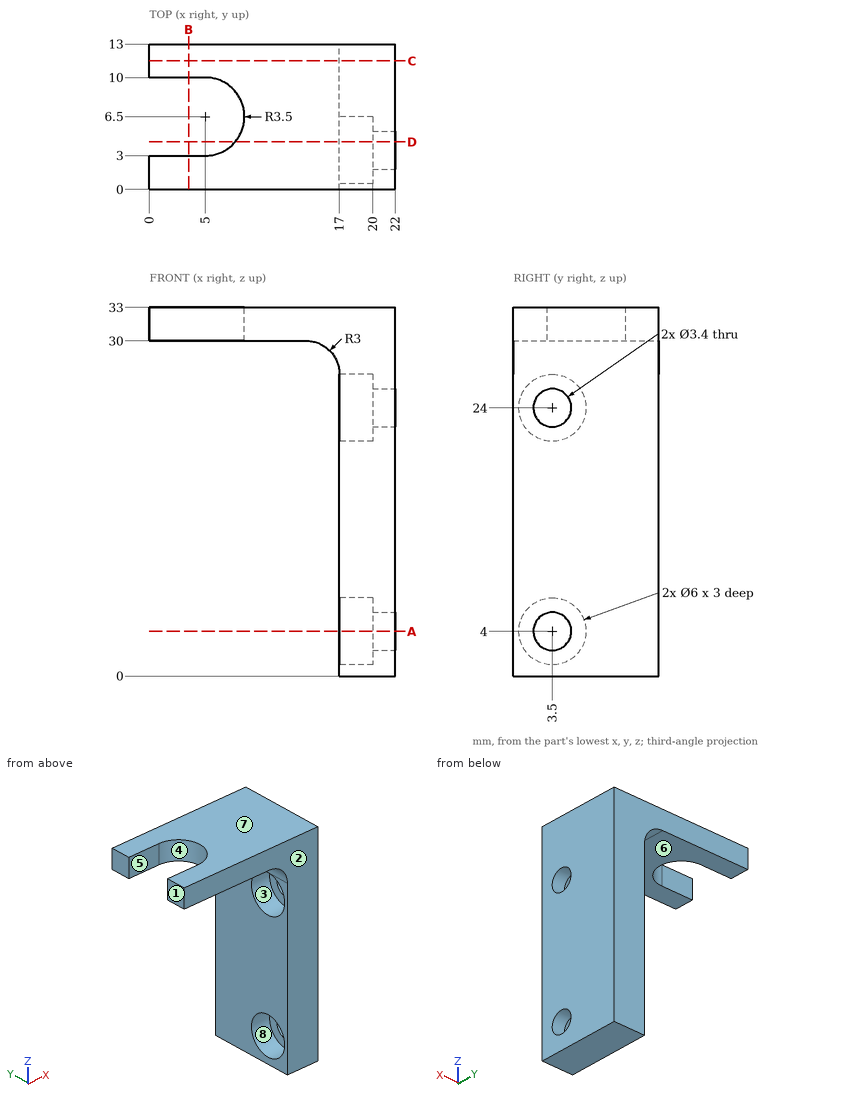
Study the drawing (mm; zero at the part's minimum x, y, z) and answer. A direction names the side the tool comes from. Coordinates: 2 decimals unless noted, no trailing zeros. Write each loop counter-clockwise with the first axis right and the second up, starting at its lowest first coordinate (ties: lowest second). Pieces come first, ordered by that corner, then holes. Notation, with made-up numbers: (-31.5, -26) - (22.5, -26) arc R23 ccw to (22.5, -17) - close; hole circle Ø6 at (81, 71.5). An arc over 180 degrees is marked (long way). Return JSON: item names as keys, results as strings. Group by question number.
1. A cutting plane is placed at C-C, the plane y = 11.5. Determine the outline of the cut face in (x, z), plus the area to 3 significant figures.
2. Straight lines are drawn through the part: L1, parallel to Y at x = 21.25, z = 4; L2, parallel to Y at x = 18.55, z = 24; L3, parallel to X at y = 4, z = 20.5. For each, find the intervals that lie inside material, in ascending order.
3. Which of the six approach directions +Z, -Z, +X, -X, +Y, -Y give full straight-line access (tool end or side, diameter ignored) to the marked faces 5, 6, 7 and 8?
4. Given pin 1 (1.8 mm diameter, centred on y = 3, z = 2.5, fed in from -X); pin 2 (4 mm diameter, centred on x = 8.5, y = 5.5, fed in from -Z); pin 3 (3.5 mm diameter, centred on x = 3, z = 31, fed in from -Y); pin 4 (5 mm diameter, centred on y = 2.5, z = 24.5, fed in from -X), each flat-ended and moving along its own axis, determine where each tip first touches the part or whether it passes through.
5. A cutting plane is placed at D-D, the plane y = 4.25. Determine the outline of the cut face in (x, z).
6. Determine the mould class of the marked faces 1, 2, 3 and 4 for opening direction Y: released by +Y, released by -Y, zero draft, split by the parting line, or undercut.
7. A cutting plane is placed at A-A, the plane z = 4. Determine the outline of the cut face in (x, y), plus the area to 3 significant figures.
8. A cutting plane is placed at B-B, the plane x = 3.5. Determine the outline of the cut face in (y, z), plus the area to 3 significant figures.
Ans:
{
 "1": {"outline": "(0, 30) - (14, 30) arc R3 cw to (17, 27) - (17, 0) - (22, 0) - (22, 33) - (0, 33) - close", "area": "218 mm²"},
 "2": {"L1": "0 to 1.8, 5.2 to 13", "L2": "0 to 0.5, 6.5 to 13", "L3": "17 to 22"},
 "3": {"face 5": "+Z, -Z, -X", "face 6": "-Z, -X, +Y, -Y", "face 7": "+Z, +X, -X, +Y, -Y", "face 8": "-X"},
 "4": {"pin 1": "x = 20", "pin 2": "z = 30", "pin 3": "y = 0", "pin 4": "x = 17"},
 "5": {"outline": "(7.68, 30) - (14, 30) arc R3 cw to (17, 27) - (17, 26.9) - (20, 26.9) - (20, 25.53) - (22, 25.53) - (22, 33) - (7.68, 33) - close; (17, 0) - (22, 0) - (22, 2.47) - (20, 2.47) - (20, 1.1) - (17, 1.1) - close; (17, 6.9) - (20, 6.9) - (20, 5.53) - (22, 5.53) - (22, 22.47) - (20, 22.47) - (20, 21.1) - (17, 21.1) - close"},
 "6": {"face 1": "zero draft", "face 2": "released by -Y", "face 3": "undercut", "face 4": "undercut"},
 "7": {"outline": "(17, 0) - (22, 0) - (22, 1.8) - (20, 1.8) - (20, 0.5) - (17, 0.5) - close; (17, 6.5) - (20, 6.5) - (20, 5.2) - (22, 5.2) - (22, 13) - (17, 13) - close", "area": "40.2 mm²"},
 "8": {"outline": "(0, 30) - (3, 30) - (3, 33) - (0, 33) - close; (10, 30) - (13, 30) - (13, 33) - (10, 33) - close", "area": "18.0 mm²"}
}
